Geometry check sheet. Reference: the model listing, model coordinates, mm. Face numbers are marked on the shaded views. A direction names the side the tool comes from. Coordinates: 2 decimals unless noted, no trailing zeros. Order: outer loops, then holes, each group sorted by start corner. A loop starts at its lowest first (then second) coordinate and runs counter-clockwise, first axis right, second up. Notation, with made-up numbers: (59.25, -9.75) - (83.25, -9.75) arc R18 ccw to (83.25, 10.25) - close; hole circle Ø3 at (68.5, -29). An arc over 180 degrees is marked (long way). Use CSV: the item, a comma, the result in double quotes. Start each with the question number.
1) Sectioned sample at C-C, the plane z = 0. Record the cut outline in (x, y), and give its area (3 significant figures).
2) Depth check by flat-ended pin: P1, Ø2, axis at x = -55, z = 35.5, coming from the +Y side. Enter the tip coordinate at first touch or a pass-through.
3) Sectioned sample at A-A, the plane x = 0. Record the cut outline in (y, z), and give its area (3 significant figures).
4) Sectioned sample at D-D, the plane x = 73. Record the cut outline in (y, z), and give its area (3 significant figures).
5) Tool access check on the marked faces 4 and 5. Record the directions out of +Z, -Z, +X, -X, +Y, -Y that give a thin tool (end or side, any length) a straight path to the whole face; none if there is none.
6) Sectioned sample at B-B, the plane y = -50. Record the cut outline in (x, z).
7) Thickness scan on probe 1 along Z at (x, y) = (0, -27); probe 2 along Y at (x, z) = (-48, 33); probe 3 along Z at (x, y) = (-16, -49). Record the ranges inside material, lowest first. Write a range as [from, to].
8) Draft check along Y on the marked faces 1, 2 and 3. Enter one of: released by +Y, released by -Y, zero draft, split by the parting line, or undercut.
from build123d import *

# Parameters (mm, degrees)
F0_W        = 200
F0_H        = 100
F1_DEPTH    = 100
F2_R        = 35.8409251955
F3_DEPTH    = 100.001
F4_R        = 5
F5_T        = -2.5
F6_T1_DEPTH = 225
F6_T3_DEPTH = 125


# Not quite as in the source:
# - a fillet or chamfer that OpenCascade refuses, or shapes differently, is made with other operations: its cross-section is extruded or revolved along the edge and cut away or added


with BuildPart() as f1:
    # F0 (on Front) → F1 (new body)
    with BuildSketch(Plane.XZ):
        Rectangle(F0_W, F0_H)
    extrude(amount=F1_DEPTH)

    # F2 (on face) → F3 (cut, through all)
    with BuildSketch(Plane.XZ.offset(100)):
        Circle(F2_R)
    extrude(amount=-F3_DEPTH, mode=Mode.SUBTRACT)

    # F4
    f4_edges = [f1.edges().sort_by_distance(p)[0] for p in [
        (-35.840925, -100, 0),
        (-35.840925, 0, 0),
    ]]
    fillet(f4_edges, radius=F4_R)

    # F5
    f5_openings = [f1.faces().sort_by_distance(p)[0] for p in [
        (0, -50, 50),
    ]]
    offset(amount=F5_T, openings=f5_openings)

    # F6: fillet of radius 5 on 4 edges, made by hand

    # F6_s2 → F6_t1 (cut)
    with BuildSketch(Plane.YZ.offset(-112.5)):
        with BuildLine():
            ThreePointArc((-100, 45), (-98.5355339059, 48.5355339059), (-95, 50))
            Line((-95, 50), (-100, 50))
            Line((-100, 50), (-100, 45))
        make_face()
        with BuildLine():
            ThreePointArc((0, 45), (-1.4644660941, 48.5355339059), (-5, 50))
            Line((-5, 50), (0, 50))
            Line((0, 50), (0, 45))
        make_face()
    extrude(amount=F6_T1_DEPTH, mode=Mode.SUBTRACT)

    # F6_s4 → F6_t3 (cut)
    with BuildSketch(Plane.XZ.offset(-12.5)):
        with BuildLine():
            ThreePointArc((-100, 45), (-98.5355339059, 48.5355339059), (-95, 50))
            Line((-95, 50), (-100, 50))
            Line((-100, 50), (-100, 45))
        make_face()
        with BuildLine():
            ThreePointArc((100, 45), (98.5355339059, 48.5355339059), (95, 50))
            Line((95, 50), (100, 50))
            Line((100, 50), (100, 45))
        make_face()
    extrude(amount=F6_T3_DEPTH, mode=Mode.SUBTRACT)


solid = f1.part
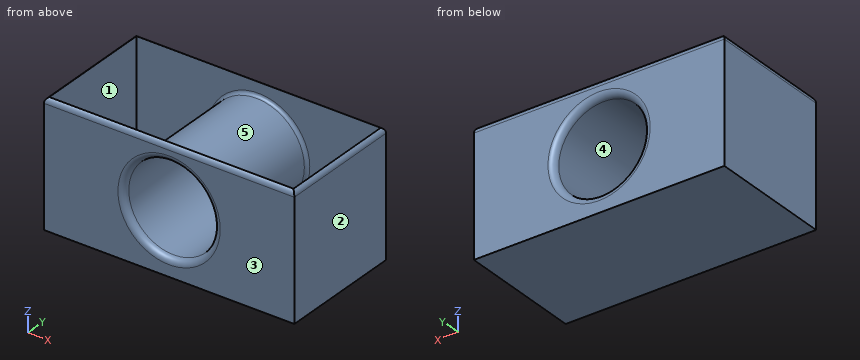
Evaluation:
1,outline,"(-100, -100) - (-40.84, -100) arc R5 ccw to (-35.84, -95) - (-35.84, -5) arc R5 ccw to (-40.84, 0) - (-100, 0) - close; (35.84, -95) arc R5 ccw to (40.84, -100) - (100, -100) - (100, 0) - (40.84, 0) arc R5 ccw to (35.84, -5) - close; hole (-97.5, -97.5) - (-40.84, -97.5) arc R2.5 ccw to (-38.34, -95) - (-38.34, -5) arc R2.5 ccw to (-40.84, -2.5) - (-97.5, -2.5) - close; hole (38.34, -95) arc R2.5 ccw to (40.84, -97.5) - (97.5, -97.5) - (97.5, -2.5) - (40.84, -2.5) arc R2.5 ccw to (38.34, -5) - close"
1,area,"1,580 mm²"
2,P1,"y = 0"
3,outline,"(-100, -50) - (0, -50) - (0, -40.84) arc R5 ccw to (-5, -35.84) - (-95, -35.84) arc R5 ccw to (-100, -40.84) - close; (-100, 40.84) arc R5 ccw to (-95, 35.84) - (-5, 35.84) arc R5 ccw to (0, 40.84) - (0, 45) arc R5 ccw to (-2.5, 49.33) - (-2.5, 40.84) arc R2.5 cw to (-5, 38.34) - (-95, 38.34) arc R2.5 cw to (-97.5, 40.84) - (-97.5, 49.33) arc R5 ccw to (-100, 45) - close; hole (-97.5, -47.5) - (-2.5, -47.5) - (-2.5, -40.84) arc R2.5 ccw to (-5, -38.34) - (-95, -38.34) arc R2.5 ccw to (-97.5, -40.84) - close"
3,area,"828 mm²"
4,outline,"(-100, -50) - (0, -50) - (0, 45) arc R5 ccw to (-2.5, 49.33) - (-2.5, -47.5) - (-97.5, -47.5) - (-97.5, 49.33) arc R5 ccw to (-100, 45) - close"
4,area,"728 mm²"
5,face 4,"+Y, -Y"
5,face 5,"none"
6,outline,"(-100, -50) - (100, -50) - (100, 45) arc R5 ccw to (97.5, 49.33) - (97.5, -47.5) - (-97.5, -47.5) - (-97.5, 49.33) arc R5 ccw to (-100, 45) - close; circle Ø76.68 at (0, 0); hole circle Ø71.68 at (0, 0)"
7,probe 1,"[-50, -47.5], [-38.34, -35.84], [35.84, 38.34]"
7,probe 2,"[-100, -97.5], [-2.5, 0]"
7,probe 3,"[-50, -47.5], [-34.84, -32.07], [32.07, 34.84]"
8,face 1,"undercut"
8,face 2,"zero draft"
8,face 3,"released by -Y"
